Source: CAD feature listing. Evaluate the final solid. Frame: model axes, mm. Face numbers are marked on the shaded views. Give positions to 0.01 mm unless a question says otherwise; leave off trailing zeros. Loops run counter-clockwise (first coordinate to the right, second up) from the corner with the lowest first, then second, coordinate; pieces in that order, holes last.
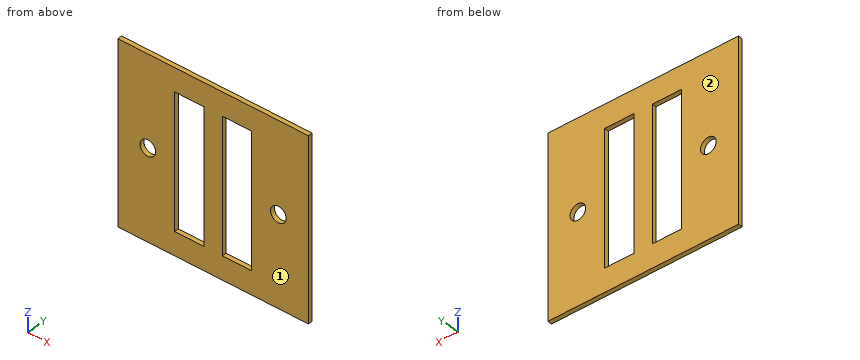
```python
from build123d import *

# Parameters (mm, degrees)
SKETCH1_W           = 130
SKETCH1_H           = 120
BOSS_EXTRUDE1_DEPTH = 3
CUT_EXTRUDE1_START  = -4
SKETCH2_W           = 20
SKETCH2_H           = 89
CUT_EXTRUDE1_DEPTH  = 5
CUT_EXTRUDE2_START  = -4
SKETCH3_R           = 5.3
CUT_EXTRUDE2_DEPTH  = 5


with BuildPart() as part:
    # Sketch1 → Boss-Extrude1 (new body)
    with BuildSketch(Plane(origin=(0, 0, 0), x_dir=(1, 0, 0), z_dir=(0, 1, 0))):
        Rectangle(SKETCH1_W, SKETCH1_H)
    extrude(amount=BOSS_EXTRUDE1_DEPTH)

    # Sketch2 → Cut-Extrude1 (cut)
    with BuildSketch(Plane(origin=(0, 3, 0), x_dir=(1, 0, 0), z_dir=(0, 1, 0)).offset(CUT_EXTRUDE1_START)):
        with Locations((-16.25, 0)):
            Rectangle(SKETCH2_W, SKETCH2_H)
    cut_extrude1 = extrude(amount=CUT_EXTRUDE1_DEPTH, mode=Mode.SUBTRACT)

    # Mirror1: Cut-Extrude1 across plane
    add(cut_extrude1.mirror(Plane(origin=(0, 0, 0), x_dir=(0, 0, 1), z_dir=(1, 0, 0))), mode=Mode.SUBTRACT)

    # Sketch3 → Cut-Extrude2 (cut)
    with BuildSketch(Plane(origin=(0, 3, 0), x_dir=(1, 0, 0), z_dir=(0, 1, 0)).offset(CUT_EXTRUDE2_START)):
        with Locations((44.5, 0)):
            Circle(SKETCH3_R)
    cut_extrude2 = extrude(amount=CUT_EXTRUDE2_DEPTH, mode=Mode.SUBTRACT)

    # Mirror2: Cut-Extrude2 across plane
    add(cut_extrude2.mirror(Plane(origin=(0, 0, 0), x_dir=(0, 0, 1), z_dir=(1, 0, 0))), mode=Mode.SUBTRACT)


solid = part.part
```
(1) Section C-C, the plane y = 2. Return the cut outline in (x, z).
A:
outline: (-65, -60) - (65, -60) - (65, 60) - (-65, 60) - close; hole circle Ø10.6 at (-44.5, 0); hole (-26.25, -44.5) - (-6.25, -44.5) - (-6.25, 44.5) - (-26.25, 44.5) - close; hole (6.25, -44.5) - (26.25, -44.5) - (26.25, 44.5) - (6.25, 44.5) - close; hole circle Ø10.6 at (44.5, 0)
(2) Mould query, pull axis Y, two halves, no side actions, for the marked faces 1 and 2. Classes: pulls with the +Y half, pulls with the -Y half, needs draft (parallel to the pull), parting line crosses it, or undercut.
A:
face 1: pulls with the -Y half
face 2: pulls with the +Y half
(3) Section B-B, the plane x = 44.5. Return the cut outline in (y, z), then the cut area to 3 significant figures.
A:
outline: (0, -60) - (3, -60) - (3, -5.3) - (0, -5.3) - close; (0, 5.3) - (3, 5.3) - (3, 60) - (0, 60) - close
area: 328 mm2
(4) Section A-A, the plane z = -34.5. Return the cut outline in (x, y), then the cut area to 3 significant figures.
A:
outline: (-65, 0) - (-26.25, 0) - (-26.25, 3) - (-65, 3) - close; (-6.25, 0) - (6.25, 0) - (6.25, 3) - (-6.25, 3) - close; (26.25, 0) - (65, 0) - (65, 3) - (26.25, 3) - close
area: 270 mm2
(5) Section D-D, the plane z = -2.5. Return the cut outline in (x, y).
A:
outline: (-65, 0) - (-49.17, 0) - (-49.17, 3) - (-65, 3) - close; (-39.83, 0) - (-26.25, 0) - (-26.25, 3) - (-39.83, 3) - close; (-6.25, 0) - (6.25, 0) - (6.25, 3) - (-6.25, 3) - close; (26.25, 0) - (39.83, 0) - (39.83, 3) - (26.25, 3) - close; (49.17, 0) - (65, 0) - (65, 3) - (49.17, 3) - close
(6) Ray query, line 1 along X through (y, z) = (1.15, -26.5); line 2 along Z through (x, y) = (44.5, 1.65); line 3 along Z through (x, y) = (22.5, 2.6). Return the intervals inside material, ascending.
A:
line 1: x = -65 to -26.25, -6.25 to 6.25, 26.25 to 65
line 2: z = -60 to -5.3, 5.3 to 60
line 3: z = -60 to -44.5, 44.5 to 60
